Design review of the part built by this model. Coordinates are the model's own, in mm. A direction names the side the tool comes from. Round coordinates to 2 decimals unless told otherwise and drop trailing zeros. Loops run counter-clockwise (first coordinate to the right, second up) from the corner with the lowest first, then second, coordinate; pieces in that order, holes last. Notation, with made-up numbers: (-38, -16.75) - (-7, -16.75) arc R34 cw to (-7, 21.25) - close; hole circle Ø10 at (80, 1.25). An arc over 180 degrees is marked (long way). Return JSON: item names as keys, results as strings. Group by question number.
from build123d import *

# Parameters (mm, degrees)
F0_R     = 6.23749
F1_DEPTH = 2.5


with BuildPart() as f1:
    # F0 (on Top) → F1 (new body, symmetric)
    with BuildSketch(Plane.XY):
        with BuildLine():
            Line((-1.591629, 17.42747), (-1.724057, 14.900591))
            ThreePointArc((-1.724057, 14.900591), (-2.035734, 14.861218), (-2.346517, 14.815325))
            ThreePointArc((-2.346517, 14.815325), (-2.656271, 14.762934), (-2.96486, 14.704068))
            Line((-2.96486, 14.704068), (-3.871655, 17.06635))
            ThreePointArc((-3.871655, 17.06635), (-5.407797, 16.643489), (-6.899114, 16.082669))
            Line((-6.899114, 16.082669), (-6.244212, 13.638542))
            ThreePointArc((-6.244212, 13.638542), (-6.528466, 13.504782), (-6.809857, 13.365098))
            ThreePointArc((-6.809857, 13.365098), (-7.088261, 13.219552), (-7.363556, 13.068207))
            Line((-7.363556, 13.068207), (-8.955955, 15.034656))
            ThreePointArc((-8.955955, 15.034656), (-10.286242, 14.157797), (-11.531265, 13.163583))
            Line((-11.531265, 13.163583), (-10.15314, 11.041456))
            ThreePointArc((-10.15314, 11.041456), (-10.382148, 10.826403), (-10.606602, 10.606602))
            ThreePointArc((-10.606602, 10.606602), (-10.826403, 10.382148), (-11.041456, 10.15314))
            Line((-11.041456, 10.15314), (-13.163583, 11.531265))
            ThreePointArc((-13.163583, 11.531265), (-14.157797, 10.286242), (-15.034656, 8.955955))
            Line((-15.034656, 8.955955), (-13.068207, 7.363556))
            ThreePointArc((-13.068207, 7.363556), (-13.219552, 7.088261), (-13.365098, 6.809857))
            ThreePointArc((-13.365098, 6.809857), (-13.504782, 6.528466), (-13.638542, 6.244212))
            Line((-13.638542, 6.244212), (-16.082669, 6.899114))
            ThreePointArc((-16.082669, 6.899114), (-16.643489, 5.407797), (-17.06635, 3.871655))
            Line((-17.06635, 3.871655), (-14.704068, 2.96486))
            ThreePointArc((-14.704068, 2.96486), (-14.762934, 2.656271), (-14.815325, 2.346517))
            ThreePointArc((-14.815325, 2.346517), (-14.861218, 2.035734), (-14.900591, 1.724057))
            Line((-14.900591, 1.724057), (-17.42747, 1.591629))
            ThreePointArc((-17.42747, 1.591629), (-17.5, 0), (-17.42747, -1.591629))
            Line((-17.42747, -1.591629), (-14.900591, -1.724057))
            ThreePointArc((-14.900591, -1.724057), (-14.861218, -2.035734), (-14.815325, -2.346517))
            ThreePointArc((-14.815325, -2.346517), (-14.762934, -2.656271), (-14.704068, -2.96486))
            Line((-14.704068, -2.96486), (-17.06635, -3.871655))
            ThreePointArc((-17.06635, -3.871655), (-16.643489, -5.407797), (-16.082669, -6.899114))
            Line((-16.082669, -6.899114), (-13.638542, -6.244212))
            ThreePointArc((-13.638542, -6.244212), (-13.504782, -6.528466), (-13.365098, -6.809857))
            ThreePointArc((-13.365098, -6.809857), (-13.219552, -7.088261), (-13.068207, -7.363556))
            Line((-13.068207, -7.363556), (-15.034656, -8.955955))
            ThreePointArc((-15.034656, -8.955955), (-14.157797, -10.286242), (-13.163583, -11.531265))
            Line((-13.163583, -11.531265), (-11.041456, -10.15314))
            ThreePointArc((-11.041456, -10.15314), (-10.826403, -10.382148), (-10.606602, -10.606602))
            ThreePointArc((-10.606602, -10.606602), (-10.382148, -10.826403), (-10.15314, -11.041456))
            Line((-10.15314, -11.041456), (-11.531265, -13.163583))
            ThreePointArc((-11.531265, -13.163583), (-10.286242, -14.157797), (-8.955955, -15.034656))
            Line((-8.955955, -15.034656), (-7.363556, -13.068207))
            ThreePointArc((-7.363556, -13.068207), (-7.088261, -13.219552), (-6.809857, -13.365098))
            ThreePointArc((-6.809857, -13.365098), (-6.528466, -13.504782), (-6.244212, -13.638542))
            Line((-6.244212, -13.638542), (-6.899114, -16.082669))
            ThreePointArc((-6.899114, -16.082669), (-5.407797, -16.643489), (-3.871655, -17.06635))
            Line((-3.871655, -17.06635), (-2.96486, -14.704068))
            ThreePointArc((-2.96486, -14.704068), (-2.656271, -14.762934), (-2.346517, -14.815325))
            ThreePointArc((-2.346517, -14.815325), (-2.035734, -14.861218), (-1.724057, -14.900591))
            Line((-1.724057, -14.900591), (-1.591629, -17.42747))
            ThreePointArc((-1.591629, -17.42747), (0, -17.5), (1.591629, -17.42747))
            Line((1.591629, -17.42747), (1.724057, -14.900591))
            ThreePointArc((1.724057, -14.900591), (2.035734, -14.861218), (2.346517, -14.815325))
            ThreePointArc((2.346517, -14.815325), (2.656271, -14.762934), (2.96486, -14.704068))
            Line((2.96486, -14.704068), (3.871655, -17.06635))
            ThreePointArc((3.871655, -17.06635), (5.407797, -16.643489), (6.899114, -16.082669))
            Line((6.899114, -16.082669), (6.244212, -13.638542))
            ThreePointArc((6.244212, -13.638542), (6.528466, -13.504782), (6.809857, -13.365098))
            ThreePointArc((6.809857, -13.365098), (7.088261, -13.219552), (7.363556, -13.068207))
            Line((7.363556, -13.068207), (8.955955, -15.034656))
            ThreePointArc((8.955955, -15.034656), (10.286242, -14.157797), (11.531265, -13.163583))
            Line((11.531265, -13.163583), (10.15314, -11.041456))
            ThreePointArc((10.15314, -11.041456), (10.382148, -10.826403), (10.606602, -10.606602))
            ThreePointArc((10.606602, -10.606602), (10.826403, -10.382148), (11.041456, -10.15314))
            Line((11.041456, -10.15314), (13.163583, -11.531265))
            ThreePointArc((13.163583, -11.531265), (14.157797, -10.286242), (15.034656, -8.955955))
            Line((15.034656, -8.955955), (13.068207, -7.363556))
            ThreePointArc((13.068207, -7.363556), (13.219552, -7.088261), (13.365098, -6.809857))
            ThreePointArc((13.365098, -6.809857), (13.504782, -6.528466), (13.638542, -6.244212))
            Line((13.638542, -6.244212), (16.082669, -6.899114))
            ThreePointArc((16.082669, -6.899114), (16.643489, -5.407797), (17.06635, -3.871655))
            Line((17.06635, -3.871655), (14.704068, -2.96486))
            ThreePointArc((14.704068, -2.96486), (14.762934, -2.656271), (14.815325, -2.346517))
            ThreePointArc((14.815325, -2.346517), (14.861218, -2.035734), (14.900591, -1.724057))
            Line((14.900591, -1.724057), (17.42747, -1.591629))
            ThreePointArc((17.42747, -1.591629), (17.5, 0), (17.42747, 1.591629))
            Line((17.42747, 1.591629), (14.900591, 1.724057))
            ThreePointArc((14.900591, 1.724057), (14.861218, 2.035734), (14.815325, 2.346517))
            ThreePointArc((14.815325, 2.346517), (14.762934, 2.656271), (14.704068, 2.96486))
            Line((14.704068, 2.96486), (17.06635, 3.871655))
            ThreePointArc((17.06635, 3.871655), (16.643489, 5.407797), (16.082669, 6.899114))
            Line((16.082669, 6.899114), (13.638542, 6.244212))
            ThreePointArc((13.638542, 6.244212), (13.504782, 6.528466), (13.365098, 6.809857))
            ThreePointArc((13.365098, 6.809857), (13.219552, 7.088261), (13.068207, 7.363556))
            Line((13.068207, 7.363556), (15.034656, 8.955955))
            ThreePointArc((15.034656, 8.955955), (14.157797, 10.286242), (13.163583, 11.531265))
            Line((13.163583, 11.531265), (11.041456, 10.15314))
            ThreePointArc((11.041456, 10.15314), (10.826403, 10.382148), (10.606602, 10.606602))
            ThreePointArc((10.606602, 10.606602), (10.382148, 10.826403), (10.15314, 11.041456))
            Line((10.15314, 11.041456), (11.531265, 13.163583))
            ThreePointArc((11.531265, 13.163583), (10.286242, 14.157797), (8.955955, 15.034656))
            Line((8.955955, 15.034656), (7.363556, 13.068207))
            ThreePointArc((7.363556, 13.068207), (7.088261, 13.219552), (6.809857, 13.365098))
            ThreePointArc((6.809857, 13.365098), (6.528466, 13.504782), (6.244212, 13.638542))
            Line((6.244212, 13.638542), (6.899114, 16.082669))
            ThreePointArc((6.899114, 16.082669), (5.407797, 16.643489), (3.871655, 17.06635))
            Line((3.871655, 17.06635), (2.96486, 14.704068))
            ThreePointArc((2.96486, 14.704068), (2.656271, 14.762934), (2.346517, 14.815325))
            ThreePointArc((2.346517, 14.815325), (2.035734, 14.861218), (1.724057, 14.900591))
            Line((1.724057, 14.900591), (1.591629, 17.42747))
            ThreePointArc((1.591629, 17.42747), (0, 17.5), (-1.591629, 17.42747))
        make_face()
        Circle(F0_R, mode=Mode.SUBTRACT)
    extrude(amount=F1_DEPTH, both=True)


solid = f1.part
Q1. For line 1 (Y direction, x = 0, z = 0.05); line 2 (Y direction, x = 11, z = -1.4); line 3 (X direction, y = -15.5, z = -1.9), list the stretches that pass through material, from the lowest coordinate up.
Q2. Add section C-C, the plane x = -9.5. State the section outline as (y, z) points.
Q3. Tool access review of faces 1 (the flat face through (3.412, -15.869, 0.035)), 2 (the flat face through (14.1, -8.2, 0)), 3 (the flat face through (3.425, 15.902, 0.035)), 4 (the flat face through (14.843, -6.567, 0.035)): name each direction out of +Z, -Z, +X, -X, +Y, -Y from which nothing blocks a thin tool from reaching the whole face with its end or side.
Q4. Add section A-A, the plane y = 0. State the section outline as (x, z) points.
Q5. Insertion check: pin 1 Ø1 at (y, z) = (-5.5, -0.5) entering from +X; pin 2 Ø1 at (y, z) = (9, -1.5) entering from +X; pin 3 Ø1 at (y, z) = (-13.5, -2) entering from -X. Each pin has a flat end and moves straight along its axis. Give the tip position at first contact, or say it passes through.
Q6. Draft analysis for pull direction X (two halves, no side actions). For faces 5 (the flat face through (-8, 0, -2.5)), 6 (the flat face through (1.66, 16.15, 0.04)), 7 (the flat face through (14.04, 8.15, 0.04)), 8 (the cylindrical face through (-17.5, 0, 0)), state which applies: pulls with the +X half, pulls with the -X half, needs draft (parallel to the pull), parting line crosses it, or undercut.
Evaluation:
{
 "1": {"line 1": "-17.5 to -6.24, 6.24 to 17.5", "line 2": "-13.61 to -12.35, -10.2 to 10.2, 12.35 to 13.61", "line 3": "-6.74 to -3.27, -1.69 to 1.69, 3.27 to 6.74"},
 "2": {"outline": "(-14.7, -2.5) - (14.7, -2.5) - (14.7, 2.5) - (-14.7, 2.5) - close"},
 "3": {"face 1": "+Z, -Z, -Y", "face 2": "+Z, -Z, +X", "face 3": "+Z, -Z, +Y", "face 4": "+Z, -Z"},
 "4": {"outline": "(-17.5, -2.5) - (-6.24, -2.5) - (-6.24, 2.5) - (-17.5, 2.5) - close; (6.24, -2.5) - (17.5, -2.5) - (17.5, 2.5) - (6.24, 2.5) - close"},
 "5": {"pin 1": "x = 16.77", "pin 2": "x = 15.03", "pin 3": "x = -11.53"},
 "6": {"face 5": "needs draft", "face 6": "undercut", "face 7": "pulls with the +X half", "face 8": "pulls with the -X half"}
}
